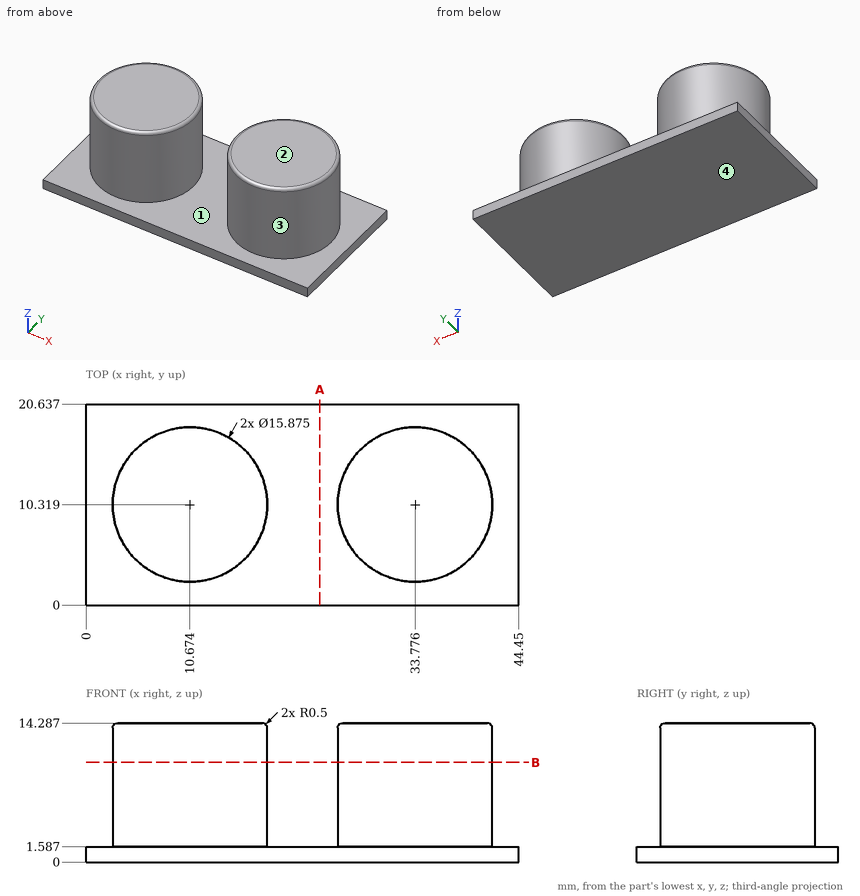
Geometry check sheet. Reference: drawing and pictorial views, mm from the part's lowest x, y, z. A direction names the side the tool comes from. Round coordinates to 2 decimals unless told otherwise and drop trailing zeros. Write each loop counter-clockwise with the first axis right and the second up, starting at its lowest first coordinate (ties: lowest second). Pieces come first, ordered by that corner, then holes.
Item 1: Material ranges on line 1 along Z through (x, y) = (40.5, 4); line 2 along X through (y, z) = (5.25, 1.75) (1 decimal); line 3 along X through (y, z) = (8.25, 8.5), recorded low to high.
Determined:
line 1: z = 0 to 1.59
line 2: x = 4.6 to 16.8, 27.7 to 39.9
line 3: x = 3.01 to 18.34, 26.11 to 41.44
Item 2: Section check A-A (x = 24). Record the boundary of the cut face in (y, z).
Determined:
outline: (0, 0) - (20.64, 0) - (20.64, 1.59) - (0, 1.59) - close
Item 3: Section check B-B (z = 10.25). Record the boundary of the cut face in (x, y) (1 decimal).
Determined:
outline: circle Ø15.9 at (10.7, 10.3); circle Ø15.9 at (33.8, 10.3)
Item 4: Mould release check, pull along X, two halves, no side actions. Record for the marked faces 1 and 2: +X half, -X half, draft (parallel to the pull), parting line (faces both ways), or undercut.
Determined:
face 1: undercut
face 2: draft
Item 5: Go/stop test with flat-tipped pins: pin 1 Ø3 at (x, z) = (11.5, 10) entering from +Y; pin 2 Ø1 at (y, z) = (10.5, 4) entering from +X; pin 3 Ø5 at (x, z) = (20.5, 8.5) entering from -Y (1 decimal). Record where each tip stops, or that it passes through.
Determined:
pin 1: stops at y = 18.26
pin 2: stops at x = 41.71
pin 3: stops at y = 7.3
Item 6: Access from +Z, -Z, +X, -X, +Y, -Y to the whole of each face (thin tool, end or side, straight path). Record for the marked faces 3 and 4.
Determined:
face 3: +Z
face 4: -Z, +X, -X, +Y, -Y
